The figure shows three views and two pictorial views of one solid part (mm, origin at its lowest corner). Answer the questions. A direction names the side the tool comes from. Give positions to 0.01 mm unless a question says otherwise; leave off trailing zeros. Loops run counter-clockwise (first coordinate to the right, second up) from the corner with the lowest first, then second, coordinate; pieces in that order, holes last. Notation, with made-up numbers: (-39.75, 80) - (2.25, 80) arc R22 ccw to (2.25, 96) - close; hole circle Ø3 at (44.25, 75). An arc over 180 degrees is marked (long way). Write item = value, one per line.
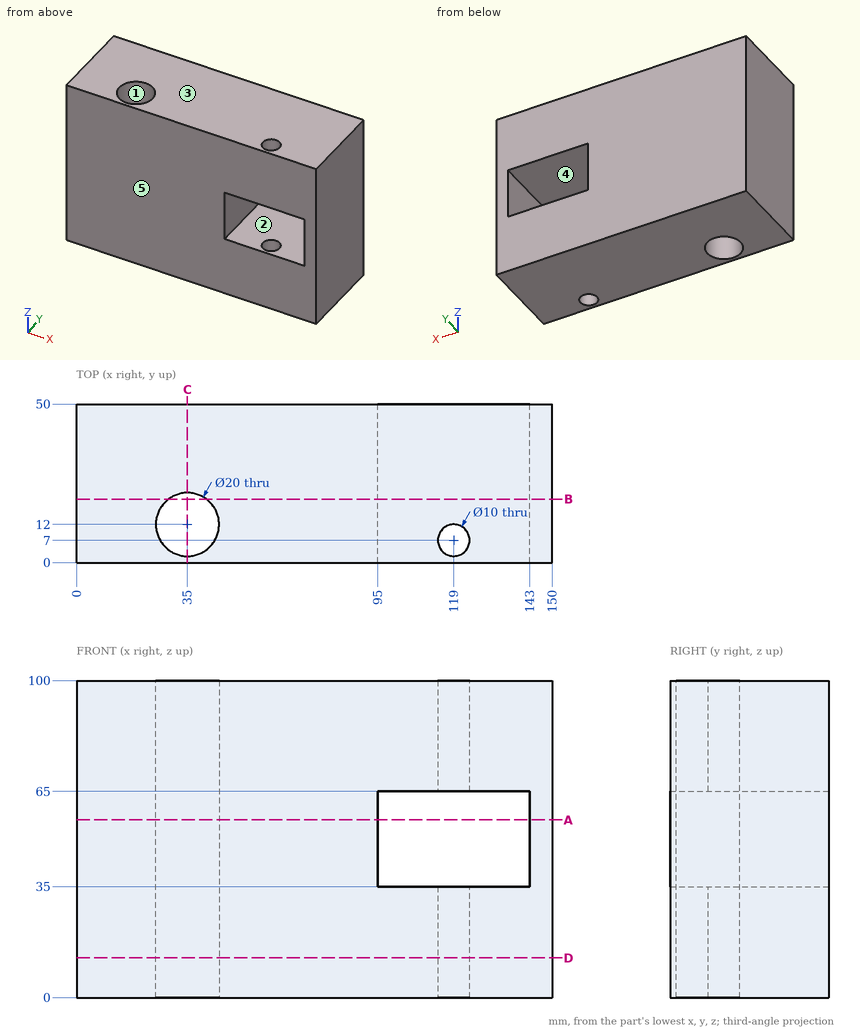
1) The mould has two halves that part along Z. Classify the marked faces 1, 2 and 3: pulls with the +Z half, pulls with the -Z half, needs draft (parallel to the pull), parting line crosses it, or undercut.
Output:
face_1 = needs draft
face_2 = undercut
face_3 = pulls with the +Z half
2) A cutting plane is placed at D-D on z = 12.5. Determine the outline of the cut face in (x, y), then the cut area to 3 significant figures.
Output:
outline = (0, 0) - (150, 0) - (150, 50) - (0, 50) - close; hole circle Ø20 at (35, 12); hole circle Ø10 at (119, 7)
area = 7,110 mm²
3) Find the intervals of material crossed by probe 1 along Y at (x, z) = (119, 21); probe 2 along X at (y, z) = (7, 25.5); probe 3 along Z at (x, y) = (123, 17), in increasing order.
Output:
probe_1 = 0 to 2, 12 to 50
probe_2 = 0 to 26.34, 43.66 to 114, 124 to 150
probe_3 = 0 to 35, 65 to 100
4) A cutting plane is placed at C-C on x = 35. Determine the outline of the cut face in (y, z), then the cut area to 3 significant figures.
Output:
outline = (0, 0) - (2, 0) - (2, 100) - (0, 100) - close; (22, 0) - (50, 0) - (50, 100) - (22, 100) - close
area = 3,000 mm²
5) A cutting plane is placed at B-B on y = 20. Determine the outline of the cut face in (x, z), then the cut area to 3 significant figures.
Output:
outline = (0, 0) - (29, 0) - (29, 100) - (0, 100) - close; (41, 0) - (150, 0) - (150, 100) - (41, 100) - close; hole (95, 35) - (143, 35) - (143, 65) - (95, 65) - close
area = 12,400 mm²
6) A tool of negligible diameter and unlimited length cuts with its end or side. For the marked faces 4 and 5, from which of +Z, -Z, +X, -X, +Y, -Y can it reach the whole face along a straight path? Write none if from no direction.
Output:
face_4 = +Y, -Y
face_5 = +Z, -Z, +X, -X, -Y
7) A cutting plane is placed at A-A on z = 56. Determine the outline of the cut face in (x, y).
Output:
outline = (0, 0) - (95, 0) - (95, 50) - (0, 50) - close; (143, 0) - (150, 0) - (150, 50) - (143, 50) - close; hole circle Ø20 at (35, 12)
